Model file for the job. Use its own axes, mm. Face numbers are marked on the shaded views. A direction names the side the tool comes from. Give positions to 0.01 mm unless a question says otherwise; leave off trailing zeros. Order: outer loops, then holes, each group sorted by start corner. A loop starts at its lowest first (then second) coordinate and runs counter-clockwise, first axis right, second up. Notation, with made-up numbers: (53, -39.75) -> (71, -39.75) arc R17 ccw to (71, -22.75) -> close; hole circle Ø4 at (-39, -21). An arc over 180 degrees is marked (long way). Use CSV: the item, a comma, the result in double quotes. Start each with the question number.
1. Cut at B-B on z = -58. List the corners of the cut face in (x, y) (3 decimals), then the cut area to 3 significant figures.
2. Drop flat-ended pins along their axis: pin 1 (8 mm diameter, centred on y = 5.5, z = -50.5, fed in from -X) (3 decimals); pin 2 (8 mm diameter, centred on x = -2, y = 4, fed in from -Z); pin 3 (12 mm diameter, centred on x = -10, z = -48.5, fed in from +Y). Give the stop position or say it passes through.
3. Cut at C-C on y = 4.5. List the corners of the cut face in (x, z) (3 decimals).
4. Pull direction Z, two halves, no side cores. Call the marked faces 1, 2 and 3: released by +Z, released by -Z, zero draft, split by the parting line, or undercut.
5. Wall check: line 1 (X direction, y = 3, z = -58) (3 decimals); line 2 (Y direction, x = 1, z = -37.5); line 3 (Z direction, x = 0, y = 6.5). Give the ranges that are in metal, low to high. Write a range as from..to.
6. 3-axis set-ups, long thin cutter, end or side, ignore diameter. For the marked faces 4, 5, 6 and 7: which of +Z, -Z, +X, -X, +Y, -Y reach the whole face in a straight line?
7. Cut at D-D on z = -31.5. List the corners of the cut face in (x, y).
8. Cut at A-A on x = 11. List the corners of the cut face in (y, z), then the cut area to 3 significant figures.
```python
from build123d import *

# Parameters (mm, degrees)
BOSS_EXTRUDE1_DEPTH  = 10
FILLET2_R            = 1
FILLET2_OF_MIRROR1_R = 1
CUT_EXTRUDE1_DEPTH   = 81.635062113
FILLET3_R            = 1
SKETCH5_R            = 2.5
BOSS_EXTRUDE2_DEPTH  = 10
FILLET1_R            = 0.5
SKETCH6_W            = 39.78759817
SKETCH6_H            = 34
CUT_EXTRUDE2_DEPTH   = 10


with BuildPart() as part:
    # Sketch2 → Boss-Extrude1 (new body)
    with BuildSketch(Plane(origin=(0, 0, 0), x_dir=(1, 0, 0), z_dir=(0, 1, 0))):
        Polygon((-19.893799085, 77.5), (0, 77.5), (0, 75.5), (-2.625, 75.5), (-2.625, 73), (-2.625, 63), (-2.625, 60.5), (0, 60.5), (0, 60.375), (0, 2.5), (-2.625, 2.5), (-2.625, 0), (-2.625, -10), (-2.625, -12.5), (0, -12.5), (0, -14.5), (-19.893799085, -14.5), align=None)
    boss_extrude1 = extrude(amount=BOSS_EXTRUDE1_DEPTH)

    # Fillet2
    fillet2_edges = [part.edges().sort_by_distance(p)[0] for p in [
        (-2.625, 5, 12.5),
        (-2.625, 5, -2.5),
        (-2.625, 5, -60.5),
        (-2.625, 5, -75.5),
    ]]
    fillet(fillet2_edges, radius=FILLET2_R)

    # Mirror1: Boss-Extrude1 across Right Plane
    add(boss_extrude1.mirror(Plane(origin=(0, 0, 0), x_dir=(0, 0, -1), z_dir=(1, 0, 0))))

    # Fillet2 of Mirror1
    fillet2_of_mirror1_edges = [part.edges().sort_by_distance(p)[0] for p in [
        (2.625, 5, 12.5),
        (2.625, 5, -2.5),
        (2.625, 5, -60.5),
        (2.625, 5, -75.5),
    ]]
    fillet(fillet2_of_mirror1_edges, radius=FILLET2_OF_MIRROR1_R)

    # Sketch4 → Cut-Extrude1 (cut, through all)
    with BuildSketch(Plane(origin=(0, 0, 0), x_dir=(1, 0, 0), z_dir=(0, 1, 0))):
        Polygon((-14.625, 15), (-14.625, 5), (-14.625, 2.5), (-12, 2.5), (-9.375, 2.5), (-9.375, 5), (-9.375, 15), (-9.375, 17.5), (-12, 17.5), (-14.625, 17.5), align=None)
        Polygon((9.375, 58), (9.375, 48), (9.375, 45.5), (12, 45.5), (14.625, 45.5), (14.625, 48), (14.625, 58), (14.625, 60.5), (12, 60.5), (9.375, 60.5), align=None)
    extrude(amount=CUT_EXTRUDE1_DEPTH, mode=Mode.SUBTRACT)

    # Fillet3
    fillet3_edges = [part.edges().sort_by_distance(p)[0] for p in [
        (-14.625, 5, -17.5),
        (-14.625, 5, -2.5),
        (-9.375, 5, -2.5),
        (-9.375, 5, -17.5),
        (14.625, 5, -60.5),
        (9.375, 5, -60.5),
        (9.375, 5, -45.5),
        (14.625, 5, -45.5),
    ]]
    fillet(fillet3_edges, radius=FILLET3_R)

    # Sketch5 → Boss-Extrude2 (add)
    with BuildSketch(Plane(origin=(0, 10, 0), x_dir=(1, 0, 0), z_dir=(0, 1, 0))):
        with Locations(Location((0, 31.5, 0), (0, 0, 90))):
            Circle(SKETCH5_R)
    extrude(amount=BOSS_EXTRUDE2_DEPTH)

    # Fillet1
    fillet1_edges = [part.edges().sort_by_distance(p)[0] for p in [
        (0, 10, -29),
    ]]
    fillet(fillet1_edges, radius=FILLET1_R)

    # Sketch6 → Cut-Extrude2 (cut)
    with BuildSketch(Plane(origin=(0, 10, 0), x_dir=(1, 0, 0), z_dir=(0, 1, 0))):
        Polygon((19.893799085, 77.5), (19.893799085, 67.609192382), (6.625, 67.609192382), (6.625, 43.5), (-6.625, 43.5), (-19.893799085, 43.5), (-19.893799085, 77.5), (-6.625, 77.5), align=None)
        with Locations((0, 2.5)):
            Rectangle(SKETCH6_W, SKETCH6_H)
    extrude(amount=-CUT_EXTRUDE2_DEPTH, mode=Mode.SUBTRACT)


solid = part.part
```
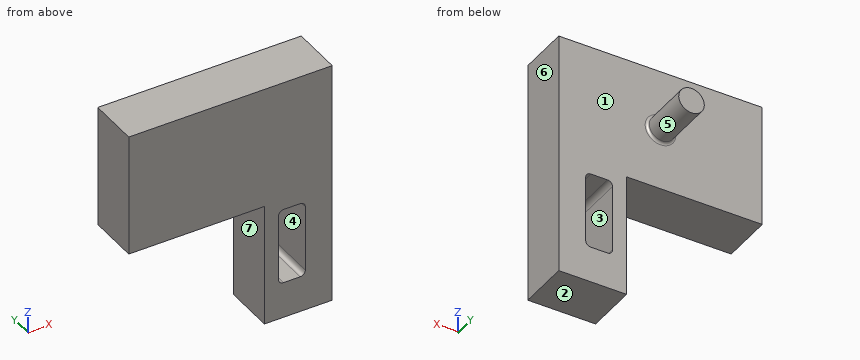
Verdict:
1,outline,"(6.625, 0) -> (9.375, 0) -> (9.375, 10) -> (6.625, 10) -> close; (14.625, 0) -> (19.894, 0) -> (19.894, 10) -> (14.625, 10) -> close"
1,area,"80.2 mm^2"
2,pin 1,"x = 6.625"
2,pin 2,"z = -43.5"
2,pin 3,"y = 10"
3,outline,"(-19.894, -43.5) -> (6.625, -43.5) -> (6.625, -67.609) -> (19.894, -67.609) -> (19.894, -19.5) -> (-19.894, -19.5) -> close; hole (9.375, -59.5) arc R1 ccw to (10.375, -60.5) -> (13.625, -60.5) arc R1 ccw to (14.625, -59.5) -> (14.625, -46.5) arc R1 ccw to (13.625, -45.5) -> (10.375, -45.5) arc R1 ccw to (9.375, -46.5) -> close"
4,face 1,"zero draft"
4,face 2,"released by -Z"
4,face 3,"undercut"
5,line 1,"6.625..9.375, 14.625..19.894"
5,line 2,"0..10"
5,line 3,"-43.5..-19.5"
6,face 4,"+Y, -Y"
6,face 5,"+Y"
6,face 6,"+Z, -Z, +X, +Y, -Y"
6,face 7,"-Z, -X, +Y, -Y"
7,outline,"(-19.89, 0) -> (19.89, 0) -> (19.89, 10) -> (3, 10) arc R0.5 cw to (2.5, 10.5) -> (2.5, 20) -> (-2.5, 20) -> (-2.5, 10.5) arc R0.5 cw to (-3, 10) -> (-19.89, 10) -> close"
8,outline,"(0, -67.61) -> (10, -67.61) -> (10, -60.5) -> (0, -60.5) -> close; (0, -45.5) -> (10, -45.5) -> (10, -19.5) -> (0, -19.5) -> close"
8,area,"331 mm^2"
